from build123d import *

# Parameters (mm, degrees)
EXTRUDE_1_DEPTH     = 8
SKETCH_2_R          = 6
EXTRUDE_2_DEPTH     = 8
SKETCH_3_R          = 2.5
CUT_EXTRUDE_1_DEPTH = 9
CHAMFER_1_SIZE      = 0.3


with BuildPart() as part:
    # 草图1 → 凸台-拉伸1 (new body)
    with BuildSketch(Plane.XY):
        with BuildLine():
            Line((-5, 0), (-5, 135))
            ThreePointArc((-5, 135), (0, 140), (5, 135))
            Line((5, 135), (5, 0))
            ThreePointArc((5, 0), (0, -5), (-5, 0))
        make_face()
    extrude(amount=EXTRUDE_1_DEPTH)

    # 草图2 → 凸台-拉伸2 (add)
    with BuildSketch(Plane.XY):
        Circle(SKETCH_2_R)
        with Locations((0, 135)):
            Circle(SKETCH_2_R)
    extrude(amount=EXTRUDE_2_DEPTH)

    # 草图3 → 切除-拉伸1 (cut, through all)
    with BuildSketch(Plane(origin=(0, 0, 0), x_dir=(-1, 0, 0), z_dir=(0, 0, -1))):
        with Locations((0, 135)):
            Circle(SKETCH_3_R)
        Circle(SKETCH_3_R)
    extrude(amount=-CUT_EXTRUDE_1_DEPTH, mode=Mode.SUBTRACT)

    # 倒角1
    chamfer_1_edges = [part.edges().sort_by_distance(p)[0] for p in [
        (5, 67.5, 0),
        (5, 67.5, 8),
        (0, -6, 8),
        (0, -6, 0),
        (-5, 67.5, 0),
        (-5, 67.5, 8),
        (0, 141, 0),
        (0, 141, 8),
        (2.5, 135, 8),
        (2.5, 135, 0),
        (2.5, 0, 8),
        (2.5, 0, 0),
    ]]
    chamfer(chamfer_1_edges, length=CHAMFER_1_SIZE)


solid = part.part
Work out the finished part from the listing and answer in its coordinate system (mm). A direction names the side the tool comes from. Round coordinates to 2 decimals unless told otherwise and drop trailing zeros. Order: outer loops, then holes, each group sorted by start corner. A loop starts at its lowest first (then second) coordinate and runs counter-clockwise, first axis right, second up. Notation, with made-up numbers: M 12,39 L 50,39 A30 ccw 50,74 Z; hole C 6.25,22.5 d11. An arc over 180 degrees is marked long. Put each result on its own line as item: value. Start each with the question number.
Q1. Section C-C, the plane z = 2.75 is taken. Write down the section's boundary in (x, y), and give its area (3 significant figures).
Q2. Section D-D, the plane y = 135 is taken. Write down the section's boundary in (x, z).
Q3. Straight lines are drawn through the part: L1, parallel to Y at x = 0, z = 3; L2, parallel to Y at x = 1.75, z = 1.75; L3, parallel to X at y = 135, z = 5.25. For each, find the intervals that lie inside material, in ascending order. Write a range as [from, to].
Q4. Section B-B, the plane x = 0 is taken. Write down the section's boundary in (y, z).
Q5. A tool of negligible diameter and unlimited length cuts with its end or side. For faces 5 (the flat face through (-5, 67, 4)), 6 (the flat face through (5, 68, 4)), 7 (the conical face through (-0.18, -5.81, 0.11)), from which of +Z, -Z, +X, -X, +Y, -Y can it reach the whole face along a straight path? Write none if from no direction.
Q6. Section A-A, the plane y = 77.5 is taken. Write down the section's boundary in (x, z), and give its area (3 significant figures).
Q7. Flat-ended cylindrical pins translate along their axes: pin 1 (3.5 mm diameter, centred on y = 66.5, z = 4.5, fed in from +X); pin 2 (1.5 mm diameter, centred on y = 86.5, z = 4.5, fed in from -X); pin 3 (1.5 mm diameter, centred on x = 3, z = 5, fed in from -Y); pin 4 (4 mm diameter, centred on x = 0, y = 135, fed in from +Z). Find the tip coordinate at first contact, or state that the pin passes through.
Q8. For a pull along X with two mould halves and no side action, classify faces 1 (the cylindrical face through (0.33, 137.48, 3.95)), 2 (the conical face through (0.18, 140.82, 7.88)), 3 (the flat face through (0, 69, 8)), 4 (the cylindrical face through (0.54, -2.44, 3.95)) as pulls with the +X half, pulls with the -X half, needs draft (parallel to the pull), parting line crosses it, or undercut.
Findings below:
1. outline: M -5,3.32 A6 ccw long 5,3.32 L 5,131.68 A6 ccw long -5,131.68 Z; hole C 0,0 d5; hole C 0,135 d5
1. area: 1,430 mm^2
2. outline: M -6,0.3 L -5.7,0 L -2.8,0 L -2.5,0.3 L -2.5,7.7 L -2.8,8 L -5.7,8 L -6,7.7 Z; M 2.5,0.3 L 2.8,0 L 5.7,0 L 6,0.3 L 6,7.7 L 5.7,8 L 2.8,8 L 2.5,7.7 Z
3. L1: y = [-6, -2.5], [2.5, 132.5], [137.5, 141]
3. L2: y = [-5.74, -1.79], [1.79, 133.21], [136.79, 140.74]
3. L3: x = [-6, -2.5], [2.5, 6]
4. outline: M -6,0.3 L -5.7,0 L -2.8,0 L -2.5,0.3 L -2.5,7.7 L -2.8,8 L -5.7,8 L -6,7.7 Z; M 2.5,0.3 L 2.8,0 L 132.2,0 L 132.5,0.3 L 132.5,7.7 L 132.2,8 L 2.8,8 L 2.5,7.7 Z; M 137.5,0.3 L 137.8,0 L 140.7,0 L 141,0.3 L 141,7.7 L 140.7,8 L 137.8,8 L 137.5,7.7 Z
5. face 5: +Z, -Z, -X
5. face 6: +Z, -Z, +X
5. face 7: -Z
6. outline: M -5,0.3 L -4.7,0 L 4.7,0 L 5,0.3 L 5,7.7 L 4.7,8 L -4.7,8 L -5,7.7 Z
6. area: 79.8 mm^2
7. pin 1: stops at x = 5
7. pin 2: stops at x = -5
7. pin 3: stops at y = -5.56
7. pin 4: passes through
8. face 1: undercut
8. face 2: parting line crosses it
8. face 3: needs draft
8. face 4: undercut
